Could you check a few things on this model? Use its own coordinates, in mm. A direction names the side the tool comes from. Round coordinates to 2 decimals unless told otherwise and drop trailing zeros. Order: outer loops, then holes, each group sorted by start corner. A loop starts at its lowest first (then second) coordinate and runs counter-clockwise, first axis right, second up. Notation, with made-up numbers: (1.25, -32.75) - (56.25, -32.75) arc R31 cw to (56.25, -2.75) - close; hole circle Ø5 at (73, 74). An arc over 180 degrees is marked (long way). Return JSON: item names as keys, results as strings. Group by question number.
from build123d import *

# Parameters (mm, degrees)
SKETCH2_W           = 71.4
SKETCH2_H           = 93
SKETCH2_W_2         = 51.4
SKETCH2_H_2         = 73
BOSS_EXTRUDE1_DEPTH = 10
SKETCH3_W           = 14
SKETCH3_H           = 26
SKETCH3_R           = 2.75
BOSS_EXTRUDE2_DEPTH = 5
SKETCH4_R           = 4
SKETCH4_R_2         = 2.75
BOSS_EXTRUDE3_DEPTH = 8.4
SKETCH5_W           = 51.4
SKETCH5_H           = 10
CUT_EXTRUDE1_DEPTH  = 65.130647899
SKETCH6_R           = 5.2
SKETCH6_R_2         = 4
BOSS_EXTRUDE4_DEPTH = 0.4
SKETCH7_W           = 71.4
SKETCH7_H           = 25
CUT_EXTRUDE2_DEPTH  = 65.130647899
FILLET1_START       = -46.5
FILLET1_DEPTH       = 5
FILLET1_2_DEPTH     = 5
SKETCH10_W          = 71.4
SKETCH10_H          = 58
CUT_EXTRUDE3_DEPTH  = 65.130647899
SKETCH9_R           = 2.55
CUT_EXTRUDE4_DEPTH  = 53.440919138
FILLET2_R           = 5
SKETCH11_R          = 2.75
BOSS_EXTRUDE5_DEPTH = 13.4
CHAMFER1_SIZE       = 0.5
CUT_EXTRUDE5_DEPTH  = 52.676783956
SKETCH14_R          = 2.1
BOSS_EXTRUDE6_DEPTH = 5
FILLET3_R           = 2


with BuildPart() as part:
    # Sketch2 → Boss-Extrude1 (new body)
    with BuildSketch(Plane(origin=(0, 0, 0), x_dir=(1, 0, 0), z_dir=(0, 1, 0))):
        Rectangle(SKETCH2_W, SKETCH2_H)
        Rectangle(SKETCH2_W_2, SKETCH2_H_2, mode=Mode.SUBTRACT)
    extrude(amount=BOSS_EXTRUDE1_DEPTH)

    # Sketch3 → Boss-Extrude2 (add)
    with BuildSketch(Plane(origin=(0, 0, -46.5), x_dir=(-1, 0, 0), z_dir=(0, 0, -1))):
        with Locations((0, 23)):
            Rectangle(SKETCH3_W, SKETCH3_H)
        with Locations((0, 30)):
            Circle(SKETCH3_R, mode=Mode.SUBTRACT)
    extrude(amount=-BOSS_EXTRUDE2_DEPTH)

    # Sketch4 → Boss-Extrude3 (add)
    with BuildSketch(Plane.XY.offset(-41.5)):
        with Locations(Location((0, 30, 0), (0, 0, 180))):
            Circle(SKETCH4_R)
        with Locations(Location((0, 30, 0), (0, 0, 180))):
            Circle(SKETCH4_R_2, mode=Mode.SUBTRACT)
    extrude(amount=BOSS_EXTRUDE3_DEPTH)

    # Sketch5 → Cut-Extrude1 (cut, through all)
    with BuildSketch(Plane(origin=(0, 10, 0), x_dir=(1, 0, 0), z_dir=(0, 1, 0))):
        with Locations((0, -41.5)):
            Rectangle(SKETCH5_W, SKETCH5_H)
    extrude(amount=-CUT_EXTRUDE1_DEPTH, mode=Mode.SUBTRACT)

    # Sketch6 → Boss-Extrude4 (add)
    with BuildSketch(Plane.XY.offset(-41.5)):
        with Locations(Location((0, 30, 0), (0, 0, 180))):
            Circle(SKETCH6_R)
        with Locations((0, 30)):
            Circle(SKETCH6_R_2, mode=Mode.SUBTRACT)
    extrude(amount=BOSS_EXTRUDE4_DEPTH)

    # Sketch7 → Cut-Extrude2 (cut, through all)
    with BuildSketch(Plane(origin=(0, 10, 0), x_dir=(1, 0, 0), z_dir=(0, 1, 0))):
        with Locations((0, -34)):
            Rectangle(SKETCH7_W, SKETCH7_H)
    extrude(amount=-CUT_EXTRUDE2_DEPTH, mode=Mode.SUBTRACT)

    # Fillet1: read off the stored shape, not the designer's step
    # Fillet1 outline → Fillet1 (cut)
    with BuildSketch(Plane.XY.offset(FILLET1_START)):
        with BuildLine():
            ThreePointArc((0, 36), (4.949747468, 33.949747468), (7, 29))
            Line((7, 29), (7, 36))
            Line((7, 36), (0, 36))
        make_face()
        with BuildLine():
            ThreePointArc((-7, 29), (-4.949747468, 33.949747468), (0, 36))
            Line((0, 36), (-7, 36))
            Line((-7, 36), (-7, 29))
        make_face()
    extrude(amount=FILLET1_DEPTH, mode=Mode.SUBTRACT)

    # Fillet1 2 outline → Fillet1 2 (add)
    with BuildSketch(Plane.XY.offset(FILLET1_START)):
        with BuildLine():
            ThreePointArc((14, 10), (9.050252532, 12.050252532), (7, 17))
            Line((7, 17), (7, 10))
            Line((7, 10), (14, 10))
        make_face()
        with BuildLine():
            Line((-14, 10), (-7, 10))
            Line((-7, 10), (-7, 17))
            ThreePointArc((-7, 17), (-9.050252532, 12.050252532), (-14, 10))
        make_face()
    extrude(amount=FILLET1_2_DEPTH)

    # Sketch10 → Cut-Extrude3 (cut, through all)
    with BuildSketch(Plane(origin=(0, 10, 0), x_dir=(1, 0, 0), z_dir=(0, 1, 0))):
        with Locations((0, 7.5)):
            Rectangle(SKETCH10_W, SKETCH10_H)
    extrude(amount=-CUT_EXTRUDE3_DEPTH, mode=Mode.SUBTRACT)

    # Sketch9 → Cut-Extrude4 (cut, through all)
    with BuildSketch(Plane(origin=(0, 0, -46.5), x_dir=(-1, 0, 0), z_dir=(0, 0, -1))):
        with Locations((-28.2, 5)):
            Circle(SKETCH9_R)
        with Locations((28.2, 5)):
            Circle(SKETCH9_R)
    extrude(amount=-CUT_EXTRUDE4_DEPTH, mode=Mode.SUBTRACT)

    # Fillet2
    fillet2_edges = [part.edges().sort_by_distance(p)[0] for p in [
        (-35.7, 10, -41.5),
        (-35.7, 0, -41.5),
        (35.7, 0, -41.5),
        (35.7, 10, -41.5),
    ]]
    fillet(fillet2_edges, radius=FILLET2_R - 0.0001)  # a hair under: the kernel refuses the full size

    # Sketch11 → Boss-Extrude5 (add)
    with BuildSketch(Plane(origin=(0, 0, -46.5), x_dir=(-1, 0, 0), z_dir=(0, 0, -1))):
        with Locations((0, 30)):
            Circle(SKETCH11_R)
        with BuildLine():
            Line((-2.05, 31.516575089), (-2.05, 28.483424911))
            ThreePointArc((-2.05, 28.483424911), (0, 27.45), (2.05, 28.483424911))
            Line((2.05, 28.483424911), (2.05, 31.516575089))
            ThreePointArc((2.05, 31.516575089), (0, 32.55), (-2.05, 31.516575089))
        make_face(mode=Mode.SUBTRACT)
    extrude(amount=-BOSS_EXTRUDE5_DEPTH)

    # Chamfer1
    chamfer1_edges = [part.edges().sort_by_distance(p)[0] for p in [
        (0, 32.55, -46.5),
        (-2.05, 30, -46.5),
        (0, 27.45, -46.5),
        (2.05, 30, -46.5),
    ]]
    chamfer(chamfer1_edges, length=CHAMFER1_SIZE)

    # Sketch12 → Cut-Extrude5 (cut, through all)
    with BuildSketch(Plane.XY.offset(-36.5)):
        with BuildLine():
            Line((-7, 17), (7, 17))
            ThreePointArc((7, 17), (9.050252532, 12.050252532), (14, 10))
            Line((14, 10), (30.7, 10))
            ThreePointArc((30.7, 10), (34.235533906, 8.535533906), (35.7, 5))
            ThreePointArc((35.7, 5), (34.235533906, 1.464466094), (30.7, 0))
            Line((30.7, 0), (-30.7, 0))
            ThreePointArc((-30.7, 0), (-34.235533906, 1.464466094), (-35.7, 5))
            ThreePointArc((-35.7, 5), (-34.235533906, 8.535533906), (-30.7, 10))
            Line((-30.7, 10), (-14, 10))
            ThreePointArc((-14, 10), (-9.050252532, 12.050252532), (-7, 17))
        make_face()
    extrude(amount=-CUT_EXTRUDE5_DEPTH, mode=Mode.SUBTRACT)


with BuildPart() as cut_extrude5_kept_piece:
    # of the separate pieces the step leaves, the one the design keeps (cut_extrude5_pieces_kept)
    add(part.part.solids().sort_by_distance((7, 17, -46.5))[0])

    # Sketch14 → Boss-Extrude6 (add)
    with BuildSketch(Plane.XY.offset(-41.5)):
        Polygon((-7, 21.5), (-7.5, 17.5), (-7.5, 11.5), (7.5, 11.5), (7.5, 17.5), (7, 21.5), (7, 17), (-7, 17), align=None)
        with Locations((-4.5, 14.5)):
            Circle(SKETCH14_R, mode=Mode.SUBTRACT)
        with Locations((4.5, 14.5)):
            Circle(SKETCH14_R, mode=Mode.SUBTRACT)
    extrude(amount=-BOSS_EXTRUDE6_DEPTH)

    # Fillet3
    fillet3_edges = [cut_extrude5_kept_piece.edges().sort_by_distance(p)[0] for p in [
        (-7.5, 17.5, -44),
        (-7.5, 11.5, -44),
        (7.5, 11.5, -44),
        (7.5, 17.5, -44),
        (7, 21.5, -44),
        (-7, 21.5, -44),
    ]]
    fillet(fillet3_edges, radius=FILLET3_R)


solid = cut_extrude5_kept_piece.part
1) I want a section at A-A, the plane y = 14.5. List the corners of the cut face in (x, z) for me.
2) I want a section at B-B, the plane z = -40.25. List the corners of the cut face in (x, y) for me.
3) I want a section at C-C, the plane z = -42.75. List the corners of the cut face in (x, y) for me.
4) For faces 4 (the conical face through (-0.04, 32.69, -46.14)), 5 (the flat face through (-7, 25, -44)), 6 (the cylindrical face through (0.521, 26.034, -37.156)), 7 (the cylindrical face through (0.03, 27.45, -39.64)), which set-ups out of +Z, -Z, +X, -X, +Y, -Y let a thin tool reach every point of the face, with its end or its side?
5) If I drill on line 1 along Z through (x, y) = (-3, 18); line 2 along Y through (x, z) = (-4.5, -45.3); line 3 along Y through (x, z) = (0.5, -45.25), over which ranges is the centre line in solid material (lowest first)? Write a range as from..to.
6) We'd pull the mould along Y, two halves only. Please class faces 1 (the flat face through (0, 24, -46.5)), 2 (the flat face through (0, 11.5, -44)), 3 (the conical face through (0.04, 27.31, -46.14)): +Y half, -Y half, draft (parallel to the pull), parting line (faces both ways), or undercut.
7) I want a section at D-D, the plane y = 30. List the corners of the cut face in (x, z) for me.
8) Will these pins go through, and if not, where does the flat tip stop? pin 1 (5 mm diameter, centred on y = 21, z = -40, fed in from +X); pin 2 (3.5 mm diameter, centred on y = 30.5, z = -41.5, fed in from -X); pin 3 (1.5 mm diameter, centred on x = -2.5, z = -44, fed in from +Y); pin 4 (2.5 mm diameter, centred on x = 4.5, y = 14.5, fed in from -Z).
Outcome:
{
 "1": {"outline": "(-7.5, -46.5) - (-6.6, -46.5) - (-6.6, -41.5) - (-7.5, -41.5) - close; (-2.4, -46.5) - (2.4, -46.5) - (2.4, -41.5) - (-2.4, -41.5) - close; (6.6, -46.5) - (7.5, -46.5) - (7.5, -41.5) - (6.6, -41.5) - close"},
 "2": {"outline": "circle Ø8 at (0, 30); hole (-2.05, 28.48) arc R2.55 ccw to (2.05, 28.48) - (2.05, 31.52) arc R2.55 ccw to (-2.05, 31.52) - close"},
 "3": {"outline": "(-7.5, 13.5) arc R2 ccw to (-5.5, 11.5) - (5.5, 11.5) arc R2 ccw to (7.5, 13.5) - (7.5, 17.38) arc R2 ccw to (7.48, 17.62) - (7.02, 21.38) arc R2 cw to (7, 21.62) - (7, 29) arc R7 ccw to (-7, 29) - (-7, 21.62) arc R2 cw to (-7.02, 21.38) - (-7.48, 17.62) arc R2 ccw to (-7.5, 17.38) - close; hole circle Ø4.2 at (-4.5, 14.5); hole (-2.05, 28.48) arc R2.55 ccw to (2.05, 28.48) - (2.05, 31.52) arc R2.55 ccw to (-2.05, 31.52) - close; hole circle Ø4.2 at (4.5, 14.5)"},
 "4": {"face 4": "-Z", "face 5": "+Z, -Z, -X, +Y", "face 6": "+Z", "face 7": "+Z, -Z"},
 "5": {"line 1": "-46.5..-41.5", "line 2": "11.5..12.4, 16.6..34.36", "line 3": "11.5..27.5, 32.5..35.98"},
 "6": {"face 1": "draft", "face 2": "-Y half", "face 3": "undercut"},
 "7": {"outline": "(-6.93, -46.5) - (-2.55, -46.5) - (-2.05, -46) - (-2.05, -33.1) - (-4, -33.1) - (-4, -41.1) - (-5.2, -41.1) - (-5.2, -41.5) - (-6.93, -41.5) - close; (2.05, -46) - (2.55, -46.5) - (6.93, -46.5) - (6.93, -41.5) - (5.2, -41.5) - (5.2, -41.1) - (4, -41.1) - (4, -33.1) - (2.05, -33.1) - close"},
 "8": {"pin 1": "x = 7.31", "pin 2": "x = -7", "pin 3": "y = 35.78", "pin 4": "through"}
}
